from build123d import *

# Parameters (mm, degrees)
SKETCH1_R           = 25
SKETCH1_R_2         = 15.625
BOSS_EXTRUDE1_DEPTH = 5
SKETCH2_R           = 18.15
CUT_EXTRUDE1_DEPTH  = 2
SKETCH3_R           = 2
CUT_EXTRUDE2_DEPTH  = 5
CUT_EXTRUDE3_DEPTH  = 2.7
BOSS_EXTRUDE2_START = 2.5
SKETCH5_R           = 2.7
SKETCH5_R_2         = 2
BOSS_EXTRUDE2_DEPTH = 2.5
FILLET1_R           = 0.5
FILLET2_R           = 0.5
FILLET3_R           = 0.5


with BuildPart() as part:
    # Sketch1 → Boss-Extrude1 (new body)
    with BuildSketch(Plane.XY):
        Circle(SKETCH1_R)
        Circle(SKETCH1_R_2, mode=Mode.SUBTRACT)
    extrude(amount=BOSS_EXTRUDE1_DEPTH)

    # Sketch2 → Cut-Extrude1 (cut)
    with BuildSketch(Plane.XY.offset(5)):
        Circle(SKETCH2_R)
    extrude(amount=-CUT_EXTRUDE1_DEPTH, mode=Mode.SUBTRACT)

    # Sketch3 → Cut-Extrude2 (cut)
    with BuildSketch(Plane.XY.offset(5)):
        with Locations((0, 21)):
            Circle(SKETCH3_R)
        with Locations((-18.186533479, -10.5)):
            Circle(SKETCH3_R)
        with Locations((18.186533479, -10.5)):
            Circle(SKETCH3_R)
    extrude(amount=-CUT_EXTRUDE2_DEPTH, mode=Mode.SUBTRACT)

    # Sketch4 → Cut-Extrude3 (cut)
    with BuildSketch(Plane(origin=(0, 0, 0), x_dir=(-1, 0, 0), z_dir=(0, 0, -1))):
        Polygon((3.464101615, 21), (1.732050808, 24), (-1.732050808, 24), (-3.464101615, 21), (-1.732050808, 18), (1.732050808, 18), align=None)
        Polygon((-16.454482672, -13.5), (-19.918584287, -13.5), (-21.650635095, -10.5), (-19.918584287, -7.5), (-16.454482672, -7.5), (-14.722431864, -10.5), align=None)
        Polygon((19.918584287, -13.5), (21.650635095, -10.5), (19.918584287, -7.5), (16.454482672, -7.5), (14.722431864, -10.5), (16.454482672, -13.5), align=None)
    extrude(amount=-CUT_EXTRUDE3_DEPTH, mode=Mode.SUBTRACT)

    # Sketch5 → Boss-Extrude2 (add)
    # profile 1 of 3: a face of its own
    with BuildSketch(Plane.XY.offset(5).offset(BOSS_EXTRUDE2_START)):
        with Locations((0, 21)):
            Circle(SKETCH5_R)
        with Locations((0, 21)):
            Circle(SKETCH5_R_2, mode=Mode.SUBTRACT)
    # profile 2 of 3: a face of its own
    with BuildSketch(Plane.XY.offset(5).offset(BOSS_EXTRUDE2_START)):
        with Locations((-18.186533479, -10.5)):
            Circle(SKETCH5_R)
        with Locations((-18.186533479, -10.5)):
            Circle(SKETCH5_R_2, mode=Mode.SUBTRACT)
    # profile 3 of 3: a face of its own
    with BuildSketch(Plane.XY.offset(5).offset(BOSS_EXTRUDE2_START)):
        with Locations((18.186533479, -10.5)):
            Circle(SKETCH5_R)
        with Locations((18.186533479, -10.5)):
            Circle(SKETCH5_R_2, mode=Mode.SUBTRACT)
    extrude(amount=-BOSS_EXTRUDE2_DEPTH)

    # Fillet1
    # the kernel refuses this fillet: 0.5 mm, written as the material it adds along each edge
    with BuildSketch(Plane(origin=(-18.186533479, -10.5, 5), x_dir=(1, 0, 0), z_dir=(0, -1, 0))) as fillet1_piece_1_section:
        with BuildLine():
            CenterArc((2.7 + FILLET1_R, FILLET1_R), FILLET1_R, 180, 90)
            Line((2.7, FILLET1_R), (2.7, 0))
            Line((2.7, 0), (2.7 + FILLET1_R, 0))
        make_face()
    fillet1_piece_1 = revolve(axis=Axis((-18.186533479, -10.5, 5), (0, 0, 1)), mode=Mode.PRIVATE)
    fillet1_piece_1 = fillet1_piece_1 - Plane(origin=(0, 0, 5.139143481), x_dir=(1, 0, 0), z_dir=(0, 0, 1)) * Cylinder(18.15, 13, mode=Mode.PRIVATE)
    add(fillet1_piece_1)

    # Fillet2
    # the kernel refuses this fillet: 0.5 mm, written as the material it adds along each edge
    with BuildSketch(Plane(origin=(18.186533479, -10.5, 5), x_dir=(1, 0, 0), z_dir=(0, -1, 0))) as fillet2_piece_1_section:
        with BuildLine():
            CenterArc((2.7 + FILLET2_R, FILLET2_R), FILLET2_R, 180, 90)
            Line((2.7, FILLET2_R), (2.7, 0))
            Line((2.7, 0), (2.7 + FILLET2_R, 0))
        make_face()
    fillet2_piece_1 = revolve(axis=Axis((18.186533479, -10.5, 5), (0, 0, 1)), mode=Mode.PRIVATE)
    fillet2_piece_1 = fillet2_piece_1 - Plane(origin=(0, 0, 5.139143483), x_dir=(1, 0, 0), z_dir=(0, 0, 1)) * Cylinder(18.15, 13, mode=Mode.PRIVATE)
    add(fillet2_piece_1)

    # Fillet3
    # the kernel refuses this fillet: 0.5 mm, written as the material it adds along each edge
    with BuildSketch(Plane(origin=(0, 21, 5), x_dir=(1, 0, 0), z_dir=(0, -1, 0))) as fillet3_piece_1_section:
        with BuildLine():
            CenterArc((2.7 + FILLET3_R, FILLET3_R), FILLET3_R, 180, 90)
            Line((2.7, FILLET3_R), (2.7, 0))
            Line((2.7, 0), (2.7 + FILLET3_R, 0))
        make_face()
    fillet3_piece_1 = revolve(axis=Axis((0, 21, 5), (0, 0, 1)), mode=Mode.PRIVATE)
    fillet3_piece_1 = fillet3_piece_1 - Plane(origin=(0, 0, 5.139143484), x_dir=(1, 0, 0), z_dir=(0, 0, 1)) * Cylinder(18.15, 13, mode=Mode.PRIVATE)
    add(fillet3_piece_1)


solid = part.part
Source: CAD feature listing. Evaluate the final solid. Frame: model axes, mm. A direction names the side the tool comes from. Coordinates: 2 decimals unless noted, no trailing zeros. Order: outer loops, then holes, each group sorted by start corner. A loop starts at its lowest first (then second) coordinate and runs counter-clockwise, first axis right, second up.
Item 1: Cut plane C-C (x = 0). Return loops of the section in (y, z) (3 decimals), plus the area to 3 significant figures.
Output values:
outline: (-25, 0) - (-15.625, 0) - (-15.625, 3) - (-18.15, 3) - (-18.15, 5) - (-25, 5) - close; (15.625, 0) - (18, 0) - (18, 2.7) - (19, 2.7) - (19, 7.5) - (18.3, 7.5) - (18.3, 5.5) arc R0.5 cw to (18.15, 5.143) - (18.15, 3) - (15.625, 3) - close; (23, 2.7) - (24, 2.7) - (24, 0) - (25, 0) - (25, 5) - (24.2, 5) arc R0.5 cw to (23.7, 5.5) - (23.7, 7.5) - (23, 7.5) - close
area: 61.8 mm2
Item 2: Pull-direction query (Y, two-part tool) for faces 4 (the face through (-0.351, 23.677, 6.514)), 5 (the face through (-20.772, -12.021, 1.331)), 6 (the face through (-18, -8, 7.5)); classes: pulls with the +Y half, pulls with the -Y half, needs draft (parallel to the pull), parting line crosses it, or undercut.
Output values:
face 4: parting line crosses it
face 5: undercut
face 6: needs draft
Item 3: First-contact query: P1, Ø2, axis at y = -4.5, z = 3.5, coming from the +X side; P2, Ø2, axis at x = 18.5, z = 2, coming from the -Y side; P3, Ø0.8, axis at x = -17.5, z = 2, coming from the -Y side. Flat tips, straight axial feed; report the tip coordinate or a pass-through.
Output values:
P1: stops at x = 24.75
P2: stops at y = -17.85
P3: stops at y = -18.24
Item 4: Cut plane D-D (z = 3.75). Return loops of the section in (x, y), plus the area to 3 significant figures.
Output values:
outline: circle Ø50 at (0, 0); hole circle Ø4 at (-18.19, -10.5); hole circle Ø36.3 at (0, 0); hole circle Ø4 at (0, 21); hole circle Ø4 at (18.19, -10.5)
area: 891 mm2
Item 5: Cut plane B-B (z = 6.5). Return loops of the section in (x, y).
Output values:
outline: circle Ø5.4 at (-18.19, -10.5); circle Ø5.4 at (0, 21); circle Ø5.4 at (18.19, -10.5); hole circle Ø4 at (-18.19, -10.5); hole circle Ø4 at (0, 21); hole circle Ø4 at (18.19, -10.5)
Item 6: Set-up query: faces 1 (the face through (23.846, 7.509, 2.465)), 2 (the face through (-18, -7.5, 1)), 3 (the face through (-15.61, -9.69, 6.51)). Return all of +Z, -Z, +X, -X, +Y, -Y with unobstructed straight access to the full face (end or side cutting, diameter ignored); none if empty.
Output values:
face 1: +Z, -Z
face 2: -Z
face 3: +Z
Item 7: Material intervals for line 1 (Y direction, x = 0, z = 1.6) (3 decimals); line 2 (Y direction, x = 0, z = 4.4); line 3 (Z direction, x = -20.5, y = -3), sorted ascending.
Output values:
line 1: y = -25 to -15.625, 15.625 to 18, 24 to 25
line 2: y = -25 to -18.15, 18.15 to 19, 23 to 25
line 3: z = 0 to 5
Item 8: Cut plane A-A (y = 0). Return loops of the section in (x, z) (3 decimals).
Output values:
outline: (-25, 0) - (-15.625, 0) - (-15.625, 3) - (-18.15, 3) - (-18.15, 5) - (-25, 5) - close; (15.625, 0) - (25, 0) - (25, 5) - (18.15, 5) - (18.15, 3) - (15.625, 3) - close
